Source: CAD feature listing. Evaluate the final solid. Frame: model axes, mm. A direction names the side the tool comes from. Round coordinates to 2 decimals unless told otherwise and drop trailing zeros. Order: outer loops, then holes, each group sorted by start corner. A loop starts at its lowest first (then second) coordinate and runs counter-clockwise, first axis right, second up. Notation, with made-up numbers: (64.25, 62) -> (102.25, 62) arc R26 cw to (102.25, 80) -> close; hole circle Ø5 at (53.25, 36.25). An arc over 180 degrees is marked (long way). Answer as CSV lines item,"result".
from build123d import *

# Parameters (mm, degrees)
F0_R     = 60.055036
F1_DEPTH = 25.4
F3_DEPTH = 12.7
F4_R     = 11.387781
F5_DEPTH = 12.7


with BuildPart() as f1:
    # F0 (on Front) → F1 (new body)
    with BuildSketch(Plane.XZ):
        with Locations((-50.623428, 0)):
            Circle(F0_R)
    extrude(amount=F1_DEPTH)

    # F2 (on face) → F3 (join)
    with BuildSketch(Plane.XZ.offset(25.4)):
        Polygon((-73.100491, 17.074037), (-67.482652, 24.497394), (-69.7838, 33.517985), (-78.271125, 37.343121), (-86.553497, 33.092397), (-88.394122, 23.966694), (-82.406971, 16.837853), align=None)
    extrude(amount=F3_DEPTH)

    # F4 (on face) → F5 (join)
    with BuildSketch(Plane.XZ.offset(25.4)):
        with Locations((-63.326038, -28.41799)):
            Circle(F4_R)
    extrude(amount=F5_DEPTH)


solid = f1.part
1. Section query D-D on y = -23. Return loops of the section in (x, z), and give its area (3 significant figures).
Results below:
outline,"circle Ø120.11 at (-50.62, 0)"
area,"11,300 mm2"
2. Line query: L1, parallel to Y at x = -92, z = -24.5; L2, parallel to X at y = -21, z = -40; L3, parallel to X at y = -27, z = 23. Output: solid intervals per line, ascending. Write a range as [from, to].
Results below:
L1,"[-25.4, 0]"
L2,"[-95.42, -5.83]"
L3,"[-87.58, -68.62]"
3. Pin query (flat end, axial travel): pin 1 (8 mm diameter, centred on x = -27, y = -25.5, fed in from +Z); pin 2 (2 mm diameter, centred on x = -17, y = -8, fed in from +Z); pin 3 (1 mm diameter, centred on x = -9.5, y = -14.5, fed in from +Z); pin 4 (3 mm diameter, centred on x = -42.5, z = -16.5, fed in from +Y). Return the tip coordinate at first contact, or that it passes through.
Results below:
pin 1,"z = 56.76"
pin 2,"z = 50.42"
pin 3,"z = 44.23"
pin 4,"y = 0"
4. Section query A-A on y = -32. Return loops of the section in (x, z).
Results below:
outline,"(-88.39, 23.97) -> (-82.41, 16.84) -> (-73.1, 17.07) -> (-67.48, 24.5) -> (-69.78, 33.52) -> (-78.27, 37.34) -> (-86.55, 33.09) -> close; circle Ø22.78 at (-63.33, -28.42)"
5. Reachability of faces 1 (the flat face through (-82.35, -31.66, 35.25)), 2 (the flat face through (-70.331, -31.661, 20.734)), 3 (the cylindrical face through (-65.795, -31.661, -39.535)), 4 (the flat face through (-73.968, -31.661, 35.404)) from +Z, -Z, +X, -X, +Y, -Y: full face, straight path, thin tool, end or side. Return the list, or none.
Results below:
face 1,"+Z, -X, -Y"
face 2,"+X, -Y"
face 3,"-Y"
face 4,"+Z, +X, -Y"
6. Section query C-C on z = 27. Return loops of the section in (x, y), and give its area (3 significant figures).
Results below:
outline,"(-104.27, -25.4) -> (-87.78, -25.4) -> (-87.78, -38.1) -> (-68.12, -38.1) -> (-68.12, -25.4) -> (3.02, -25.4) -> (3.02, 0) -> (-104.27, 0) -> close"
area,"2,970 mm2"
7. Section query B-B on x = -66. Return loops of the section in (y, z), and give its area (3 significant figures).
Results below:
outline,"(-38.1, -39.49) -> (-25.4, -39.49) -> (-25.4, -58.05) -> (0, -58.05) -> (0, 58.05) -> (-25.4, 58.05) -> (-25.4, -17.35) -> (-38.1, -17.35) -> close"
area,"3,230 mm2"
